```python
from build123d import *

# Parameters (mm, degrees)
SKETCH1_W               = 57.45
SKETCH1_H               = 80
CUT_EXTRUDE1_DEPTH      = 58.45
CUT_EXTRUDE1_DEPTH_BACK = 58.45
SKETCH3_R               = 10
CUT_EXTRUDE3_DEPTH      = 81.0000001


with BuildPart() as part:
    # Sketch1 → Revolve2 (revolve)
    with BuildSketch(Plane(origin=(0, 0, 0), x_dir=(1, 0, 0), z_dir=(0, 1, 0))):
        with Locations((28.725, 0)):
            Rectangle(SKETCH1_W, SKETCH1_H)
    revolve(axis=Axis((0, 0, 40), (0, 0, -1)))

    # Sketch2 → Cut-Extrude1 (cut, two sides)
    with BuildSketch(Plane(origin=(0, 0, 0), x_dir=(1, 0, 0), z_dir=(0, 1, 0))) as cut_extrude1_sk:
        with BuildLine():
            Line((-18.006693033, 40), (-57.45, 40))
            Line((-57.45, 40), (-57.45, -40))
            Line((-57.45, -40), (-16.882331675, -40))
            ThreePointArc((-16.882331675, -40), (-34.014765262, -0.232886901), (-18.006693033, 40))
        make_face()
    extrude(amount=CUT_EXTRUDE1_DEPTH, mode=Mode.SUBTRACT)
    extrude(cut_extrude1_sk.sketch, amount=-CUT_EXTRUDE1_DEPTH_BACK, mode=Mode.SUBTRACT)

    # Sketch3 → Cut-Extrude3 (cut, through all)
    with BuildSketch(Plane.XY.offset(40)):
        with Locations((-6.882331675, 0)):
            Circle(SKETCH3_R)
    extrude(amount=-CUT_EXTRUDE3_DEPTH, mode=Mode.SUBTRACT)


solid = part.part
```
The listing builds one solid part. Answer for the finished solid, in the listing's coordinates (mm). Coordinates: 2 decimals unless noted, no trailing zeros. Loops run counter-clockwise (first coordinate to the right, second up) from the corner with the lowest first, then second, coordinate; pieces in that order, holes last. Notation, with made-up numbers: (-28, -27.5) -> (-10, -27.5) arc R29 cw to (-10, -2.5) -> close; hole circle Ø1 at (67.5, -16.75). An arc over 180 degrees is marked (long way). Use one line per item in the form item = value. Start each with the question number.
Item 1: The part is cut by section B-B on z = 34.5. Determine the outline of the cut face in (x, y).
Item 2: The part is cut by section A-A on x = 0. Determine the outline of the cut face in (y, z), then the cut area to 3 significant figures.
Item 3: The mould has two halves that part along X. Classify faces 1 (the face through (2.656, 3.004, 0.56)), 2 (the face through (13, -1, 40)), 3 (the face through (-34, 1, 1)), 4 (the face through (57.423, 1.773, -0.56)): released by +X, released by -X, zero draft, split by the parting line, or undercut.
Item 4: Consider L1, parallel to X at y = 9, z = -0.5; L2, parallel to X at y = 5, z = -28.5; L3, parallel to Y at x = -11.5, z = -8. Determine where each line is inside the solid, lowest interval first. Write a range as [from, to].
Item 5: The part is cut by section C-C on y = -38. Determine the outline of the cut face in (x, z), then the cut area to 3 significant figures.
Item 6: The part is cut by section D-D on x = 20. Determine the outline of the cut face in (y, z).
Item 7: Flat-ended cylindrical pins translate along their axes: pin 1 Ø1.5 at (y, z) = (-5, 19.5) entering from +X; pin 2 Ø10 at (x, z) = (30.5, 16.5) entering from -Y; pin 3 Ø10 at (x, z) = (21, -7) entering from +Y. Find the tip coordinate at first contact, or state that the pin passes through.
Answer key:
q1.outline = (-21.84, -53.14) arc R57.45 ccw (long way) to (-21.84, 53.14) -> close; hole circle Ø20 at (-6.88, 0)
q2.outline = (-57.45, -40) -> (-7.25, -40) -> (-7.25, 40) -> (-57.45, 40) -> close; (7.25, -40) -> (57.45, -40) -> (57.45, 40) -> (7.25, 40) -> close
q2.area = 8,030 mm2
q3.face_1 = undercut
q3.face_2 = zero draft
q3.face_3 = released by -X
q3.face_4 = split by the parting line
q4.L1 = [-34.02, -11.24], [-2.52, 56.74]
q4.L2 = [-26.64, -15.54], [1.78, 57.23]
q4.L3 = [-56.29, -8.87], [8.87, 56.29]
q5.outline = (-18.01, -40) -> (43.09, -40) -> (43.09, 40) -> (-16.88, 40) arc R56.57 ccw to start
q5.area = 5,760 mm2
q6.outline = (-53.86, -40) -> (53.86, -40) -> (53.86, 40) -> (-53.86, 40) -> close
q7.pin_1 = 57.29
q7.pin_2 = -51.48
q7.pin_3 = 55.18
